from build123d import *

# Parameters (mm, degrees)
SKETCH1_W                      = 40
SKETCH1_H                      = 2428
BASE_FLANGE1_DEPTH             = 2
EDGE_FLANGE1_STRIP_W           = 13
EDGE_FLANGE1_STRIP_H           = 2
EDGE_FLANGE1_STRIP_CUT_DEPTH   = 2428
EDGE_FLANGE1_STRIP_2_W         = 13
EDGE_FLANGE1_STRIP_2_H         = 2
EDGE_FLANGE1_STRIP_CUT_2_DEPTH = 2428
EDGE_FLANGE1_DEPTH             = 2428
EDGE_FLANGE1_BEND_DEPTH        = 2428
EDGE_FLANGE2_STRIP_W           = 13
EDGE_FLANGE2_STRIP_H           = 2
EDGE_FLANGE2_STRIP_CUT_DEPTH   = 2428
EDGE_FLANGE2_STRIP_2_W         = 13
EDGE_FLANGE2_STRIP_2_H         = 2
EDGE_FLANGE2_STRIP_CUT_2_DEPTH = 2428
EDGE_FLANGE2_DEPTH             = 2428
EDGE_FLANGE2_BEND_DEPTH        = 2428


# Sheet-metal steps are written as plain solids
with BuildPart() as part:
    # Sketch1 → Base-Flange1 (new body)
    with BuildSketch(Plane.XY):
        Rectangle(SKETCH1_W, SKETCH1_H)
    extrude(amount=-BASE_FLANGE1_DEPTH)

    # Edge-Flange1 strip (across the edge) → Edge-Flange1 strip cut (cut)
    with BuildSketch(Plane(origin=(20, 1214, -2), x_dir=(-1, 0, 0), z_dir=(0, -1, 0))):
        with Locations((-2, -1)):
            Rectangle(EDGE_FLANGE1_STRIP_W, EDGE_FLANGE1_STRIP_H)
    extrude(amount=EDGE_FLANGE1_STRIP_CUT_DEPTH, mode=Mode.SUBTRACT)

    # Edge-Flange1 strip 2 (across the edge) → Edge-Flange1 strip cut 2 (cut)
    with BuildSketch(Plane(origin=(-20, -1214, -2), x_dir=(1, 0, 0), z_dir=(0, 1, 0))):
        with Locations((-2, -1)):
            Rectangle(EDGE_FLANGE1_STRIP_2_W, EDGE_FLANGE1_STRIP_2_H)
    extrude(amount=EDGE_FLANGE1_STRIP_CUT_2_DEPTH, mode=Mode.SUBTRACT)

    # Edge-Flange1 section (across the edge) → Edge-Flange1 (add)
    with BuildSketch(Plane(origin=(20, 1214, -2), x_dir=(-1, 0, 0), z_dir=(0, -1, 0))):
        with BuildLine():
            Line((0, 2.5), (0, 38))
            Line((0, 38), (2, 38))
            Line((2, 38), (2, 2.5))
            ThreePointArc((2, 2.5), (2.732233047, 0.732233047), (4.5, 0))
            Line((4.5, 0), (4.5, -2))
            ThreePointArc((4.5, -2), (1.318019485, -0.681980515), (0, 2.5))
        make_face()
    extrude(amount=EDGE_FLANGE1_DEPTH)

    # Edge-Flange1 section 2 (across the edge) → Edge-Flange1 bend (add)
    with BuildSketch(Plane(origin=(-20, -1214, -2), x_dir=(1, 0, 0), z_dir=(0, 1, 0))):
        with BuildLine():
            Line((0, 2.5), (0, 38))
            Line((0, 38), (2, 38))
            Line((2, 38), (2, 2.5))
            ThreePointArc((2, 2.5), (2.732233047, 0.732233047), (4.5, 0))
            Line((4.5, 0), (4.5, -2))
            ThreePointArc((4.5, -2), (1.318019485, -0.681980515), (0, 2.5))
        make_face()
    extrude(amount=EDGE_FLANGE1_BEND_DEPTH)

    # Edge-Flange2 strip (across the edge) → Edge-Flange2 strip cut (cut)
    with BuildSketch(Plane(origin=(-20, 1214, -40), x_dir=(0, 0, 1), z_dir=(0, -1, 0))):
        with Locations((-2, -1)):
            Rectangle(EDGE_FLANGE2_STRIP_W, EDGE_FLANGE2_STRIP_H)
    extrude(amount=EDGE_FLANGE2_STRIP_CUT_DEPTH, mode=Mode.SUBTRACT)

    # Edge-Flange2 strip 2 (across the edge) → Edge-Flange2 strip cut 2 (cut)
    with BuildSketch(Plane(origin=(20, -1214, -40), x_dir=(0, 0, 1), z_dir=(0, 1, 0))):
        with Locations((-2, -1)):
            Rectangle(EDGE_FLANGE2_STRIP_2_W, EDGE_FLANGE2_STRIP_2_H)
    extrude(amount=EDGE_FLANGE2_STRIP_CUT_2_DEPTH, mode=Mode.SUBTRACT)

    # Edge-Flange2 section (across the edge) → Edge-Flange2 (add)
    with BuildSketch(Plane(origin=(-20, 1214, -40), x_dir=(0, 0, 1), z_dir=(0, -1, 0))):
        with BuildLine():
            Line((0, 2.5), (0, 28))
            Line((0, 28), (2, 28))
            Line((2, 28), (2, 2.5))
            ThreePointArc((2, 2.5), (2.732233047, 0.732233047), (4.5, 0))
            Line((4.5, 0), (4.5, -2))
            ThreePointArc((4.5, -2), (1.318019485, -0.681980515), (0, 2.5))
        make_face()
    extrude(amount=EDGE_FLANGE2_DEPTH)

    # Edge-Flange2 section 2 (across the edge) → Edge-Flange2 bend (add)
    with BuildSketch(Plane(origin=(20, -1214, -40), x_dir=(0, 0, 1), z_dir=(0, 1, 0))):
        with BuildLine():
            Line((0, 2.5), (0, 28))
            Line((0, 28), (2, 28))
            Line((2, 28), (2, 2.5))
            ThreePointArc((2, 2.5), (2.732233047, 0.732233047), (4.5, 0))
            Line((4.5, 0), (4.5, -2))
            ThreePointArc((4.5, -2), (1.318019485, -0.681980515), (0, 2.5))
        make_face()
    extrude(amount=EDGE_FLANGE2_BEND_DEPTH)


solid = part.part
Verification items for the finished model (mm, model axes). Give positions to 0.01 mm unless a question says otherwise; leave off trailing zeros. Write each loop counter-clockwise with the first axis right and the second up, starting at its lowest first coordinate (ties: lowest second). Pieces come first, ordered by that corner, then holes. Notation, with made-up numbers: (-36, 39.5) -> (12, 39.5) arc R20 cw to (12, 57.5) -> close; hole circle Ø2 at (-23.75, -25.5). An arc over 180 degrees is marked (long way). Use CSV: the item, a comma, the result in double quotes.
(1) Go/stop test with flat-tipped pins: pin 1 (12 mm diameter, centred on y = -160.5, z = -18.5, fed in from -X); pin 2 (15.5 mm diameter, centred on y = 334.5, z = -15, fed in from +X); pin 3 (8 mm diameter, centred on y = -657, z = -33, fed in from +X). Record where each tip stops, or that it passes through.
Derived:
pin 1,"stops at x = -20"
pin 2,"stops at x = 20"
pin 3,"stops at x = 20.5"
(2) Sectioned sample at A-A (z = -29.5). Record the cut outline in (x, y).
Derived:
outline,"(-20, -1214) -> (-18, -1214) -> (-18, 1214) -> (-20, 1214) -> close; (18, -1214) -> (20, -1214) -> (20, 1214) -> (18, 1214) -> close"
(3) Sectioned sample at B-B (y = -875.5). Record the cut outline in (x, z).
Derived:
outline,"(-48, -40) -> (-22.5, -40) arc R4.5 ccw to (-18, -35.5) -> (-18, -4.5) arc R2.5 cw to (-15.5, -2) -> (15.5, -2) arc R2.5 cw to (18, -4.5) -> (18, -35.5) arc R4.5 ccw to (22.5, -40) -> (48, -40) -> (48, -38) -> (22.5, -38) arc R2.5 cw to (20, -35.5) -> (20, -4.5) arc R4.5 ccw to (15.5, 0) -> (-15.5, 0) arc R4.5 ccw to (-20, -4.5) -> (-20, -35.5) arc R2.5 cw to (-22.5, -38) -> (-48, -38) -> close"
(4) Material ranges on L1, parallel to X at y = 22.5, z = -33; L2, parallel to Z at x = -15, y = -917.5; L3, parallel to Z at x = 33.5, y = -530, recorded low to high.
Derived:
L1,"x = -20 to -18, 18 to 20"
L2,"z = -2 to 0"
L3,"z = -40 to -38"
